Verification items for this drawing (mm, ordinates from the low corner). Coordinates: 2 decimals unless noted, no trailing zeros. Write each loop counter-clockwise with the first axis right and the second up, starting at its lowest first coordinate (ties: lowest second). Pieces come first, ordered by that corner, then holes. Notation, with made-up numbers: M 85.5,-25.5 L 115.5,-25.5 A16 ccw 115.5,-15.5 Z; hole C 24,33 d6. An arc over 180 degrees is marked long. Answer as CSV lines item,"result". Start each with the question number.
1) Draft check along X on the marked faces 1, 2, 3 and 4. Enter one of: +X half, -X half, draft (parallel to the pull), parting line (faces both ways), or undercut.
2) Go/stop test with flat-tipped pins: pin 1 Ø4 at (x, z) = (11.5, 11.5) entering from +Y; pin 2 Ø1.5 at (x, z) = (26, 12) entering from -Y; pin 3 Ø1.1 at (y, z) = (0.5, 26) entering from -X. Record where each tip stops, or that it passes through.
3) Section check C-C (y = 3.75). Record the cut outline in (x, z).
4) Material ranges on L1, parallel to X at y = 4, z = 15; L2, parallel to X at y = 2.25, z = 3.1 (1 decimal), recorded low to high. Write a range as [from, to].
5) Section check D-D (x = 23.25). Record the cut outline in (y, z), and give its area (3 significant figures).
6) Section check A-A (x = 15). Record the cut outline in (y, z).
7) Section check B-B (z = 15). Record the cut outline in (x, y), and give its area (3 significant figures).
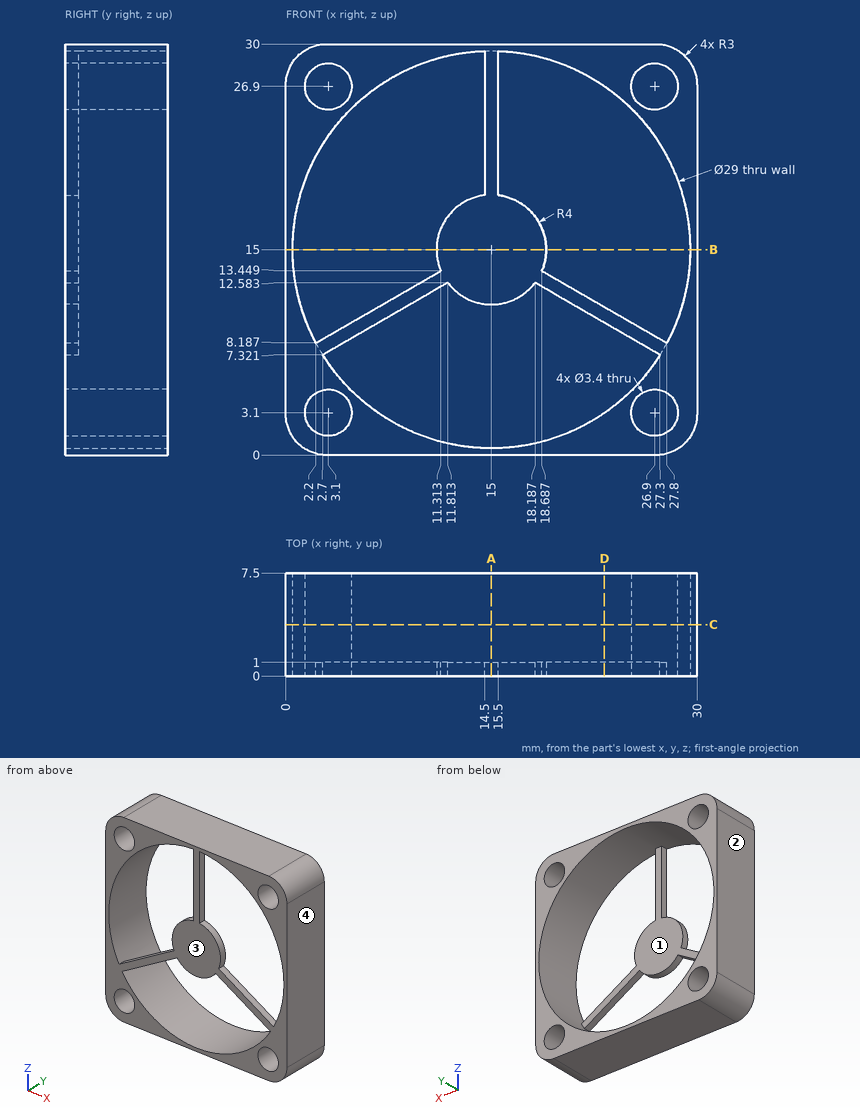
Results found:
1,face 1,"undercut"
1,face 2,"-X half"
1,face 3,"draft"
1,face 4,"+X half"
2,pin 1,"stops at y = 1"
2,pin 2,"passes through"
2,pin 3,"stops at x = 0"
3,outline,"M 0,3 A3 ccw 3,0 L 27,0 A3 ccw 30,3 L 30,27 A3 ccw 27,30 L 3,30 A3 ccw 0,27 Z; hole C 15,15 d29; hole C 3.1,3.1 d3.4; hole C 3.1,26.9 d3.4; hole C 26.9,3.1 d3.4; hole C 26.9,26.9 d3.4"
4,L1,"x = [0, 0.5], [29.5, 30]"
4,L2,"x = [0, 1.4], [4.8, 6.7], [23.3, 25.2], [28.6, 30]"
5,outline,"M 0,0 L 7.5,0 L 7.5,3.08 L 0,3.08 Z; M 0,9.66 L 1,9.66 L 1,10.81 L 0,10.81 Z; M 0,26.92 L 7.5,26.92 L 7.5,30 L 0,30 Z"
5,area,"47.3 mm2"
6,outline,"M 0,0 L 7.5,0 L 7.5,0.5 L 0,0.5 Z; M 0,11 L 1,11 L 1,29.5 L 7.5,29.5 L 7.5,30 L 0,30 Z"
7,outline,"M 0,0 L 0.5,0 L 0.5,7.5 L 0,7.5 Z; M 11,0 L 19,0 L 19,1 L 11,1 Z; M 29.5,0 L 30,0 L 30,7.5 L 29.5,7.5 Z"
7,area,"15.5 mm2"
